from build123d import *
from build123d.topology import SkipClean

# Parameters (mm, degrees)
SKETCH1_R                = 75
BOSS_EXTRUDE1_DEPTH      = 52
BOSS_EXTRUDE2_DEPTH      = 89
SKETCH6_R                = 67.5
CUT_EXTRUDE1_DEPTH       = 40
SKETCH7_R                = 10
CUT_EXTRUDE2_DEPTH       = 140
BOSS_EXTRUDE3_DEPTH      = 50
SKETCH27_R               = 13.264650289
SKETCH27_R_2             = 8.484923144
CUT_EXTRUDE7_DEPTH       = 32
SKETCH28_W               = 110.347797284
SKETCH28_H               = 32
CUT_EXTRUDE9_DEPTH       = 112
SKETCH30_R               = 1.75
CUT_EXTRUDE10_DEPTH      = 10
SKETCH31_W               = 17.16689537
SKETCH31_H               = 79.570672492
CUT_EXTRUDE11_DEPTH      = 7
SKETCH32_W               = 3
SKETCH32_H               = 75.570672492
CUT_EXTRUDE12_DEPTH      = 8.6
CUT_EXTRUDE13_START      = -8
SKETCH34_R               = 14.5
CUT_EXTRUDE13_DEPTH      = 8
BOSS_EXTRUDE4_START      = 10
SKETCH35_R               = 75
SKETCH35_R_2             = 67.5
BOSS_EXTRUDE4_DEPTH      = 10
SKETCH37_R               = 72.25
SKETCH37_R_2             = 67.5
CUT_EXTRUDE15_DEPTH      = 50
CUT_EXTRUDE16_DEPTH      = 7
CUT_EXTRUDE17_DEPTH      = 7
CUT_EXTRUDE19_REACH      = 184.003
CUT_EXTRUDE19_END_RADIUS = 72.25
SKETCH42_W               = 10
SKETCH42_H               = 42.845008339
CIRPATTERN1_COUNT        = 5
CIRPATTERN1_ANGLE        = 180
CIRPATTERN2_COUNT        = 3
CIRPATTERN2_ANGLE        = 120
CUT_EXTRUDE20_DEPTH      = 10
SKETCH44_W               = 50
SKETCH44_H               = 57
CUT_EXTRUDE21_DEPTH      = 183.002747343


with BuildPart() as part:
    # Sketch1 → Boss-Extrude1 (new body)
    with BuildSketch(Plane.XY):
        Circle(SKETCH1_R)
    extrude(amount=BOSS_EXTRUDE1_DEPTH)

    # Sketch5 → Boss-Extrude2 (add)
    with BuildSketch(Plane(origin=(0, 0, 0), x_dir=(0, 0, -1), z_dir=(1, 0, 0))):
        Polygon((-52, 59.314332163), (-52, 0), (-52, -59.3), (-47, -59.3), (-47, 59.314332163), align=None)
    extrude(amount=BOSS_EXTRUDE2_DEPTH)

    # Sketch6 → Cut-Extrude1 (cut)
    with BuildSketch(Plane(origin=(0, 0, 0), x_dir=(-1, 0, 0), z_dir=(0, 0, -1))):
        Circle(SKETCH6_R)
    extrude(amount=-CUT_EXTRUDE1_DEPTH, mode=Mode.SUBTRACT)

    # Sketch7 → Cut-Extrude2 (cut)
    with BuildSketch(Plane(origin=(0, 0, 40), x_dir=(-1, 0, 0), z_dir=(0, 0, -1))):
        Circle(SKETCH7_R)
    extrude(amount=-CUT_EXTRUDE2_DEPTH, mode=Mode.SUBTRACT)

    # Sketch8 → Boss-Extrude3 (add)
    with BuildSketch(Plane(origin=(0, 0, 40), x_dir=(-1, 0, 0), z_dir=(0, 0, -1))):
        with BuildLine():
            Line((0, 14.5), (0, 19))
            ThreePointArc((0, 19), (-19, 0), (0, -19))
            Line((0, -19), (0, -14.5))
            ThreePointArc((0, -14.5), (-14.5, 0), (0, 14.5))
        make_face()
    extrude(amount=BOSS_EXTRUDE3_DEPTH)

    # Sketch27 → Cut-Extrude7 (cut)
    with BuildSketch(Plane.XY.offset(52)):
        with Locations((-50.154049213, 0)):
            Circle(SKETCH27_R)
        with Locations((-25.142941415, 0)):
            Circle(SKETCH27_R_2)
    extrude(amount=-CUT_EXTRUDE7_DEPTH, mode=Mode.SUBTRACT)

    # Sketch28 → Cut-Extrude9 (cut)
    with BuildSketch(Plane(origin=(0, 0, 0), x_dir=(0, 0, -1), z_dir=(1, 0, 0))):
        with Locations((25.439488733, 0)):
            Rectangle(SKETCH28_W, SKETCH28_H)
    extrude(amount=-CUT_EXTRUDE9_DEPTH, mode=Mode.SUBTRACT)

    # Sketch30 → Cut-Extrude10 (cut)
    with BuildSketch(Plane(origin=(-75, 0, 0), x_dir=(0, 0, -1), z_dir=(1, 0, 0))):
        with Locations(Location((-37.43856487, -14, 0), (0, 0, 180))):
            Circle(SKETCH30_R)
    cut_extrude10 = extrude(amount=CUT_EXTRUDE10_DEPTH, mode=Mode.SUBTRACT)

    # Mirror1: Cut-Extrude10 across plane
    add(cut_extrude10.mirror(Plane.ZX), mode=Mode.SUBTRACT)

    # Sketch31 → Cut-Extrude11 (cut)
    with BuildSketch(Plane(origin=(0, 0, 40), x_dir=(-1, 0, 0), z_dir=(0, 0, -1))):
        with Locations((23.137999933, 1.261486271)):
            Rectangle(SKETCH31_W, SKETCH31_H)
    extrude(amount=-CUT_EXTRUDE11_DEPTH, mode=Mode.SUBTRACT)

    # Sketch32 → Cut-Extrude12 (cut)
    with BuildSketch(Plane.ZY.offset(14.554552248)):
        with Locations((45.5, 1.261486271)):
            Rectangle(SKETCH32_W, SKETCH32_H)
    extrude(amount=-CUT_EXTRUDE12_DEPTH, mode=Mode.SUBTRACT)

    # Sketch34 → Cut-Extrude13 (cut)
    with SkipClean():  # the faces are left unmerged after this step: merging them gives an invalid solid
        with BuildSketch(Plane(origin=(0, 0, 40), x_dir=(-1, 0, 0), z_dir=(0, 0, -1)).offset(CUT_EXTRUDE13_START)):
            with Locations(Location((0, 0, 0), (0, 0, 90))):
                Circle(SKETCH34_R)
        extrude(amount=CUT_EXTRUDE13_DEPTH, mode=Mode.SUBTRACT)

    # Sketch35 → Boss-Extrude4 (add)
    with BuildSketch(Plane(origin=(0, 0, 0), x_dir=(-1, 0, 0), z_dir=(0, 0, -1)).offset(BOSS_EXTRUDE4_START)):
        Circle(SKETCH35_R)
        Circle(SKETCH35_R_2, mode=Mode.SUBTRACT)
    extrude(amount=-BOSS_EXTRUDE4_DEPTH)

    # Sketch37 → Cut-Extrude15 (cut)
    with BuildSketch(Plane(origin=(0, 0, -10), x_dir=(-1, 0, 0), z_dir=(0, 0, -1))):
        Circle(SKETCH37_R)
        Circle(SKETCH37_R_2, mode=Mode.SUBTRACT)
    extrude(amount=-CUT_EXTRUDE15_DEPTH, mode=Mode.SUBTRACT)

    # Sketch38 → Cut-Extrude16 (cut)
    with BuildSketch(Plane(origin=(0, 0, 40), x_dir=(-1, 0, 0), z_dir=(0, 0, -1))):
        with BuildLine():
            Line((0, -23), (68.491331568, -23))
            ThreePointArc((68.491331568, -23), (-72.25, 0), (68.491331568, 23))
            Line((68.491331568, 23), (0, 23))
            ThreePointArc((0, 23), (-23, 0), (0, -23))
        make_face()
    extrude(amount=-CUT_EXTRUDE16_DEPTH, mode=Mode.SUBTRACT)

    # Sketch39 → Cut-Extrude17 (cut)
    with BuildSketch(Plane(origin=(0, 0, 40), x_dir=(-1, 0, 0), z_dir=(0, 0, -1))):
        with BuildLine():
            Line((68.491331568, 23), (31.721447618, 23))
            Line((31.721447618, 23), (31.721447618, -23))
            Line((31.721447618, -23), (68.491331568, -23))
            ThreePointArc((68.491331568, -23), (72.25, 0), (68.491331568, 23))
        make_face()
    extrude(amount=-CUT_EXTRUDE17_DEPTH, mode=Mode.SUBTRACT)

    # Cut-Extrude19: up to this cylinder (the profile starts outside it)
    cut_extrude19_end = Plane(origin=(0, 0, 11.422504), z_dir=(0, 0, -1)) * Cylinder(CUT_EXTRUDE19_END_RADIUS, 513.506, mode=Mode.PRIVATE)
    # Sketch42 → Cut-Extrude19 (cut, up to the surface)
    with BuildSketch(Plane(origin=(0, 75, 0), x_dir=(1, 0, 0), z_dir=(0, 1, 0)), mode=Mode.PRIVATE) as cut_extrude19_sk1:
        with Locations((-5, -11.42250417)):
            Rectangle(SKETCH42_W, SKETCH42_H)
    cut_extrude19_tool1 = extrude(cut_extrude19_sk1.sketch, amount=-CUT_EXTRUDE19_REACH, mode=Mode.PRIVATE) - cut_extrude19_end
    cut_extrude19 = cut_extrude19_tool1.solids().sort_by_distance((-5, 75, 11.422504))[0]
    add(cut_extrude19, mode=Mode.SUBTRACT)

    # CirPattern1: Cut-Extrude19 ×5 about axis
    cirpattern1_axis = Axis((0, 0, 0), (0, 0, -1))
    for i in range(1, CIRPATTERN1_COUNT):
        add(cut_extrude19.rotate(cirpattern1_axis, i * CIRPATTERN1_ANGLE / (CIRPATTERN1_COUNT - 1)), mode=Mode.SUBTRACT)

    # CirPattern2: Cut-Extrude19 ×3 about axis
    cirpattern2_axis = Axis((0, 0, 0), (0, 0, 1))
    for i in range(1, CIRPATTERN2_COUNT):
        add(cut_extrude19.rotate(cirpattern2_axis, i * CIRPATTERN2_ANGLE / (CIRPATTERN2_COUNT - 1)), mode=Mode.SUBTRACT)

    # Sketch43 → Cut-Extrude20 (cut)
    with BuildSketch(Plane.XY.offset(52)):
        Polygon((-45.9, -12.56399668), (-25.142941415, -8.484923144), (-25.142941415, 8.484923144), (-45.9, 12.56399668), align=None)
    extrude(amount=-CUT_EXTRUDE20_DEPTH, mode=Mode.SUBTRACT)

    # Sketch44 → Cut-Extrude21 (cut, through all)
    with SkipClean():  # the faces are left unmerged after this step: merging them gives an invalid solid
        with BuildSketch(Plane(origin=(0, 75, 0), x_dir=(1, 0, 0), z_dir=(0, 1, 0))):
            with Locations((50, -18.5)):
                Rectangle(SKETCH44_W, SKETCH44_H)
        extrude(amount=-CUT_EXTRUDE21_DEPTH, mode=Mode.SUBTRACT)
    add(part.part.scale(1), mode=Mode.REPLACE)  # the faces are merged on a copy


solid = part.part
Read the model definition and answer for the solid it produces. Units are mm, in the model's axes. A direction names the side the tool comes from. Give positions to 0.01 mm unless a question says otherwise; leave off trailing zeros. Write each loop counter-clockwise with the first axis right and the second up, starting at its lowest first coordinate (ties: lowest second). Pieces come first, ordered by that corner, then holes. Notation, with made-up numbers: (-20, 38) - (33, 38) arc R34 cw to (33, 74) - close; hole circle Ø10 at (-2, 53). An arc over 180 degrees is marked (long way). Use CSV: the item, a comma, the result in double quotes. Start each with the question number.
Item 1: For faces 4 (the flat face through (-6, -23, 43)), 5 (the flat face through (10, 3, 48)), 6 (the flat face through (67, 59.314, 49)), 7 (the cylindrical face through (-72.28, -14.08, 35.69)), 8 (the flat face through (67, -59.3, 50)), determine the directions among +Z, -Z, +X, -X, +Y, -Y from which every point of the face is accessible in a straight line to the end or side of a thin tool.
Item 2: The part is cut by section C-C, the plane x = -8. Give the vertices of the cut face in (y, z) (3 decimals), and give its area (3 significant figures).
Item 3: The part is cut by section A-A, the plane z = 15. Give the vertices of the cut face in (x, y) (3 decimals), and give its area (3 significant figures).
Item 4: The mould has two halves that part along X. Classify faces 1 (the cylindrical face through (19, 0, 15)), 2 (the cylindrical face through (-63.414, 0.352, 49.535)), 3 (the flat face through (-32, -65, -10)): pulls with the +X half, pulls with the -X half, needs draft (parallel to the pull), parting line crosses it, or undercut.
Item 5: Flat-ended cylindrical pins translate along their axes: P1, Ø2, axis at y = -17.5, z = 24, coming from the -X side; P2, Ø4.5, axis at x = -13, y = -33, coming from the -Z side; P3, Ø1, axis at x = 5, z = 0, coming from the -Y side. Find the tip coordinate at first contact, or state that the pin passes through.
Item 6: Consider line 1 (Z direction, x = -71.8, y = -14); line 2 (Y direction, x = 7.5, z = 35.5); line 3 (Z direction, x = -7, y = -14). Determine where each line is inside the solid, lowest interval first.
Item 7: The part is cut by section D-D, the plane y = -48. Give the vertices of the cut face in (x, z), and give its area (3 significant figures).
Item 8: The part is cut by section B-B, the plane x = -50.5. Give the vertices of the cut face in (y, z), and give its area (3 significant figures).
Taken from the geometry:
1,face 4,"-Z, +X"
1,face 5,"-Z"
1,face 6,"+Z, -Z, +X, +Y"
1,face 7,"-X"
1,face 8,"+Z, -Z, +X, -Y"
2,outline,"(-74.572, -10) - (-71.806, -10) - (-71.806, 47) - (-12.093, 47) - (-12.093, 48) - (-6, 48) - (-6, 52) - (-74.572, 52) - close; (-23, 40) - (-12.093, 40) - (-12.093, 44) - (-23, 44) - close; (6, 48) - (12.093, 48) - (12.093, 47) - (71.806, 47) - (71.806, 32.845) - (74.572, 32.845) - (74.572, 52) - (6, 52) - close; (12.093, 40) - (23, 40) - (23, 44) - (12.093, 44) - close"
2,area,"958 mm2"
3,outline,"(-73.273, -16) arc R75 ccw to (-64.952, -37.5) - (-62.57, -36.125) arc R72.25 cw to (-70.456, -16) - close; (-73.273, 16) - (-70.456, 16) arc R72.25 cw to (-66.968, 27.117) - (-69.372, 28.505) arc R75 ccw to start; (-64.952, 37.5) - (-62.57, 36.125) arc R72.25 cw to (-10, 71.555) - (-10, 74.33) arc R75 ccw to start; (-59.372, -45.825) arc R75 ccw to (0, -75) - (0, -72.25) arc R72.25 cw to (-56.968, -44.438) - close; (0, -19) arc R19 ccw to (0, 19) - (0, 14.5) arc R14.5 cw to (0, -14.5) - close; (0, 72.25) arc R72.25 cw to (25, 67.787) - (25, 70.711) arc R75 ccw to (0, 75) - close; (10, -74.33) arc R75 ccw to (25, -70.711) - (25, -67.787) arc R72.25 cw to (10, -71.555) - close"
3,area,"814 mm2"
4,face 1,"pulls with the +X half"
4,face 2,"undercut"
4,face 3,"needs draft"
5,P1,"x = -73.16"
5,P2,"z = 47"
5,P3,"y = -18.46"
6,line 1,"-10 to 0, 29.73 to 35.69, 39.19 to 52"
6,line 2,"-74.62 to -71.86, -17.46 to -12.41, 12.41 to 17.46, 71.86 to 74.62"
6,line 3,"40 to 44, 47 to 52"
7,outline,"(-57.63, -10) - (-54, -10) - (-54, 47) - (89, 47) - (89, 52) - (-57.63, 52) - close"
7,area,"940 mm2"
8,outline,"(-55.45, -10) - (-51.67, -10) - (-51.67, 47) - (-13.26, 47) - (-13.26, 52) - (-55.45, 52) - close; (13.26, 47) - (51.67, 47) - (51.67, -10) - (55.45, -10) - (55.45, 52) - (13.26, 52) - close"
8,area,"853 mm2"
